from build123d import *

# Parameters (mm, degrees)
HEXALOBULAR_REACH = 10.439


with BuildPart() as part:
    # BodySke → Base-Revolve (revolve)
    with BuildSketch(Plane(origin=(0, 0, 0), x_dir=(0, 0, -1), z_dir=(1, 0, 0)), mode=Mode.PRIVATE) as base_revolve_sk:
        Polygon((0, 0), (0, 1.9), (0.3, 1.9), (1.2, 1), (8, 1), (8, 0), align=None)
    revolve(base_revolve_sk.sketch.rotate(Axis((0, 0, 0), (0, 0, 1)), 90), axis=Axis((0, 0, 0), (0, 0, 1)))

    # PreBSke → PreBroach (revolve, cut)
    with BuildSketch(Plane(origin=(0, 0, 0), x_dir=(0, 0, -1), z_dir=(1, 0, 0)), mode=Mode.PRIVATE) as prebroach_sk:
        Polygon((0, 0), (0, 0.875), (0.64, 0.875), (1.165753042, 0), align=None)
    revolve(prebroach_sk.sketch.rotate(Axis((0, 0, 0), (0, 0, 1)), 90), axis=Axis((0, 0, 0), (0, 0, 1)), mode=Mode.SUBTRACT)

    # Hexalobular: up to this cone (the profile starts inside it)
    hexalobular_end = Plane(origin=(0, 0, 0), z_dir=(0, 0, 1)).offset(-1.165752042) * Cone(1.664e-06, 23.374625438, 14.04489091, align=(Align.CENTER, Align.CENTER, Align.MIN), mode=Mode.PRIVATE)
    # HexSke → Hexalobular (add, up to the surface)
    with BuildSketch(Plane.XY, mode=Mode.PRIVATE) as hexalobular_sk1:
        with BuildLine():
            ThreePointArc((-0.757772228, -0.4375), (-0.779371934, -0.324649655), (-0.726328785, -0.222727273))
            ThreePointArc((-0.726328785, -0.222727273), (-0.630273039, 0), (-0.726328785, 0.222727273))
            ThreePointArc((-0.726328785, 0.222727273), (-0.779371934, 0.324649655), (-0.757772228, 0.4375))
            ThreePointArc((-0.757772228, 0.4375), (-0.875, 0), (-0.757772228, -0.4375))
        make_face()
    hexalobular_tool1 = extrude(hexalobular_sk1.sketch, amount=-HEXALOBULAR_REACH, mode=Mode.PRIVATE) & hexalobular_end
    add(hexalobular_tool1.solids().sort_by_distance((-0.76612, 0, 0))[0])
    # HexSke → Hexalobular (add, up to the surface)
    with BuildSketch(Plane.XY, mode=Mode.PRIVATE) as hexalobular_sk2:
        with BuildLine():
            ThreePointArc((0, 0.875), (-0.4375, 0.757772228), (-0.757772228, 0.4375))
            ThreePointArc((-0.757772228, 0.4375), (-0.670840815, 0.512631066), (-0.556051869, 0.517655543))
            ThreePointArc((-0.556051869, 0.517655543), (-0.31513652, 0.545832463), (-0.170276916, 0.740382816))
            ThreePointArc((-0.170276916, 0.740382816), (-0.108531118, 0.837280721), (0, 0.875))
        make_face()
    hexalobular_tool2 = extrude(hexalobular_sk2.sketch, amount=-HEXALOBULAR_REACH, mode=Mode.PRIVATE) & hexalobular_end
    add(hexalobular_tool2.solids().sort_by_distance((-0.38306, 0.66348, 0))[0])
    # HexSke → Hexalobular (add, up to the surface)
    with BuildSketch(Plane.XY, mode=Mode.PRIVATE) as hexalobular_sk3:
        with BuildLine():
            ThreePointArc((0.757772228, 0.4375), (0.4375, 0.757772228), (0, 0.875))
            ThreePointArc((0, 0.875), (0.108531118, 0.837280721), (0.170276916, 0.740382816))
            ThreePointArc((0.170276916, 0.740382816), (0.31513652, 0.545832463), (0.556051869, 0.517655543))
            ThreePointArc((0.556051869, 0.517655543), (0.670840815, 0.512631066), (0.757772228, 0.4375))
        make_face()
    hexalobular_tool3 = extrude(hexalobular_sk3.sketch, amount=-HEXALOBULAR_REACH, mode=Mode.PRIVATE) & hexalobular_end
    add(hexalobular_tool3.solids().sort_by_distance((0.38306, 0.66348, 0))[0])
    # HexSke → Hexalobular (add, up to the surface)
    with BuildSketch(Plane.XY, mode=Mode.PRIVATE) as hexalobular_sk4:
        with BuildLine():
            ThreePointArc((0.726328785, -0.222727273), (0.779371934, -0.324649655), (0.757772228, -0.4375))
            ThreePointArc((0.757772228, -0.4375), (0.845185098, -0.226466664), (0.875, 0))
            ThreePointArc((0.875, 0), (0.845185098, 0.226466664), (0.757772228, 0.4375))
            ThreePointArc((0.757772228, 0.4375), (0.779371934, 0.324649655), (0.726328785, 0.222727273))
            ThreePointArc((0.726328785, 0.222727273), (0.630273039, 0), (0.726328785, -0.222727273))
        make_face()
    hexalobular_tool4 = extrude(hexalobular_sk4.sketch, amount=-HEXALOBULAR_REACH, mode=Mode.PRIVATE) & hexalobular_end
    add(hexalobular_tool4.solids().sort_by_distance((0.76612, 0, 0))[0])
    # HexSke → Hexalobular (add, up to the surface)
    with BuildSketch(Plane.XY, mode=Mode.PRIVATE) as hexalobular_sk5:
        with BuildLine():
            ThreePointArc((0.170276916, -0.740382816), (0.108531118, -0.837280721), (0, -0.875))
            ThreePointArc((0, -0.875), (0.4375, -0.757772228), (0.757772228, -0.4375))
            ThreePointArc((0.757772228, -0.4375), (0.670840815, -0.512631066), (0.556051869, -0.517655543))
            ThreePointArc((0.556051869, -0.517655543), (0.31513652, -0.545832463), (0.170276916, -0.740382816))
        make_face()
    hexalobular_tool5 = extrude(hexalobular_sk5.sketch, amount=-HEXALOBULAR_REACH, mode=Mode.PRIVATE) & hexalobular_end
    add(hexalobular_tool5.solids().sort_by_distance((0.38306, -0.66348, 0))[0])
    # HexSke → Hexalobular (add, up to the surface)
    with BuildSketch(Plane.XY, mode=Mode.PRIVATE) as hexalobular_sk6:
        with BuildLine():
            ThreePointArc((-0.556051869, -0.517655543), (-0.670840815, -0.512631066), (-0.757772228, -0.4375))
            ThreePointArc((-0.757772228, -0.4375), (-0.4375, -0.757772228), (0, -0.875))
            ThreePointArc((0, -0.875), (-0.108531118, -0.837280721), (-0.170276916, -0.740382816))
            ThreePointArc((-0.170276916, -0.740382816), (-0.31513652, -0.545832463), (-0.556051869, -0.517655543))
        make_face()
    hexalobular_tool6 = extrude(hexalobular_sk6.sketch, amount=-HEXALOBULAR_REACH, mode=Mode.PRIVATE) & hexalobular_end
    add(hexalobular_tool6.solids().sort_by_distance((-0.38306, -0.66348, 0))[0])

    # ThdSchSke → ThreadSchematic (revolve, cut)
    with BuildSketch(Plane(origin=(0, 0, 0), x_dir=(0, 0, -1), z_dir=(1, 0, 0))):
        Polygon((8.130481161, 1), (8, 0.774), (7.869518839, 1), align=None)
    revolve(axis=Axis((0, 0, 0), (0, 0, 1)), mode=Mode.SUBTRACT)


solid = part.part
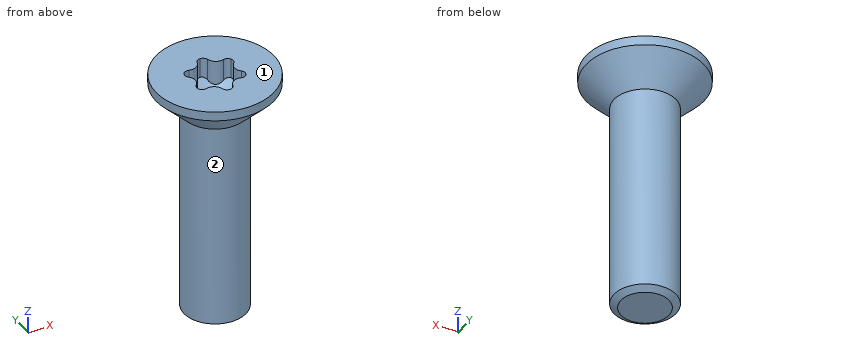
Work out the finished part from the listing and answer in its coordinate system (mm). Face numbers are marked on the shaded views. A direction names the side the tool comes from. Round coordinates to 2 decimals unless told otherwise and drop trailing zeros. Write each loop counter-clockwise with the first axis right and the second up, starting at its lowest first coordinate (ties: lowest second). Pieces come first, ordered by that corner, then holes. Notation, with made-up numbers: M 74.25,-3 L 85.25,-3 A16 cw 85.25,6 Z; hole C 13.25,-38.5 d2. An arc over 180 degrees is marked long. Use a Markdown table: item, result.
1) Which of the six approach directions +Z, -Z, +X, -X, +Y, -Y give full straight-line access (tool end or side, diameter ignored) to the marked faces 1 and 2?
Taken from the geometry:
| item | result |
|---|---|
| face 1 | +Z, +X, -X, +Y, -Y |
| face 2 | -Z |
2) Flat-ended cylindrical pins translate along their axes: pin 1 (1.5 mm diameter, centred on y = 0.5, z = -3.5, fed in from +X); pin 2 (1 mm diameter, centred on y = -1, z = -7, fed in from +X); pin 3 (1.5 mm diameter, centred on y = -1, z = -5.5, fed in from -X). Find the tip coordinate at first contact, or state that the pin passes through.
Taken from the geometry:
| item | result |
|---|---|
| pin 1 | stops at x = 1 |
| pin 2 | stops at x = 0.87 |
| pin 3 | stops at x = -0.97 |
3) The part is cut by section B-B on z = -3.25. Give the vertices of the cut face in (x, y), plus the area to 3 significant figures.
Taken from the geometry:
| item | result |
|---|---|
| outline | C 0,0 d2 |
| area | 3.14 mm2 |
4) Consider line 1 (Y direction, x = 0.7, z = -0.25); line 2 (X direction, y = 0.9, z = -3.5); line 3 (X direction, y = 0.45, z = -0.25). Determine where each line is inside the solid, lowest interval first. Write a range as [from, to].
Taken from the geometry:
| item | result |
|---|---|
| line 1 | y = [-1.77, -0.5], [-0.19, 0.19], [0.5, 1.77] |
| line 2 | x = [-0.44, 0.44] |
| line 3 | x = [-1.85, -0.75], [0.75, 1.85] |
